from build123d import *

# Parameters (mm, degrees)
SKETCH1_R           = 52.3875
SKETCH1_R_2         = 50.8
BOSS_EXTRUDE1_DEPTH = 7.9
CUT_EXTRUDE1_START  = 3.95
SKETCH1_3_R         = 52.3875
SKETCH1_3_R_2       = 50.8
CUT_EXTRUDE1_DEPTH  = 1.7653


with BuildPart() as part:
    # Sketch1 → Boss-Extrude1 (new body)
    with BuildSketch(Plane(origin=(0, 0, 0), x_dir=(1, 0, 0), z_dir=(0, 1, 0))):
        with Locations(Location((0, 0, 0), (0, 0, 270))):
            Circle(SKETCH1_R)
        Circle(SKETCH1_R_2, mode=Mode.SUBTRACT)
        Circle(SKETCH1_R_2)
        with BuildLine():
            Line((-2.54, 4.028623369), (-2.54, 45.967377631))
            ThreePointArc((-2.54, 45.967377631), (-32.553428439, 32.553428439), (-45.967377631, 2.54))
            Line((-45.967377631, 2.54), (-4.028623369, 2.54))
            ThreePointArc((-4.028623369, 2.54), (-3.367596045, 3.367596045), (-2.54, 4.028623369))
        make_face(mode=Mode.SUBTRACT)
        with BuildLine():
            Line((4.028623369, 2.54), (45.967377631, 2.54))
            ThreePointArc((45.967377631, 2.54), (32.553428439, 32.553428439), (2.54, 45.967377631))
            Line((2.54, 45.967377631), (2.54, 4.028623369))
            ThreePointArc((2.54, 4.028623369), (3.367596045, 3.367596045), (4.028623369, 2.54))
        make_face(mode=Mode.SUBTRACT)
        with BuildLine():
            Line((2.54, -4.028623369), (2.54, -45.967377631))
            ThreePointArc((2.54, -45.967377631), (32.553428439, -32.553428439), (45.967377631, -2.54))
            Line((45.967377631, -2.54), (4.028623369, -2.54))
            ThreePointArc((4.028623369, -2.54), (3.367596045, -3.367596045), (2.54, -4.028623369))
        make_face(mode=Mode.SUBTRACT)
        with BuildLine():
            ThreePointArc((2.01246118, -1.8), (2.7, 0), (2.01246118, 1.8))
            Line((2.01246118, 1.8), (-2.01246118, 1.8))
            ThreePointArc((-2.01246118, 1.8), (-2.7, 0), (-2.01246118, -1.8))
            Line((-2.01246118, -1.8), (2.01246118, -1.8))
        make_face(mode=Mode.SUBTRACT)
        with BuildLine():
            ThreePointArc((-45.967377631, -2.54), (-32.553428439, -32.553428439), (-2.54, -45.967377631))
            Line((-2.54, -45.967377631), (-2.54, -4.028623369))
            ThreePointArc((-2.54, -4.028623369), (-3.367596045, -3.367596045), (-4.028623369, -2.54))
            Line((-4.028623369, -2.54), (-45.967377631, -2.54))
        make_face(mode=Mode.SUBTRACT)
    extrude(amount=BOSS_EXTRUDE1_DEPTH)

    # Sketch1<3> → Cut-Extrude1 (cut, symmetric)
    with BuildSketch(Plane(origin=(0, 0, 0), x_dir=(1, 0, 0), z_dir=(0, 1, 0)).offset(CUT_EXTRUDE1_START)):
        with Locations(Location((0, 0, 0), (0, 0, 270))):
            Circle(SKETCH1_3_R)
        with Locations(Location((0, 0, 0), (0, 0, 270))):
            Circle(SKETCH1_3_R_2, mode=Mode.SUBTRACT)
    extrude(amount=CUT_EXTRUDE1_DEPTH, both=True, mode=Mode.SUBTRACT)


solid = part.part
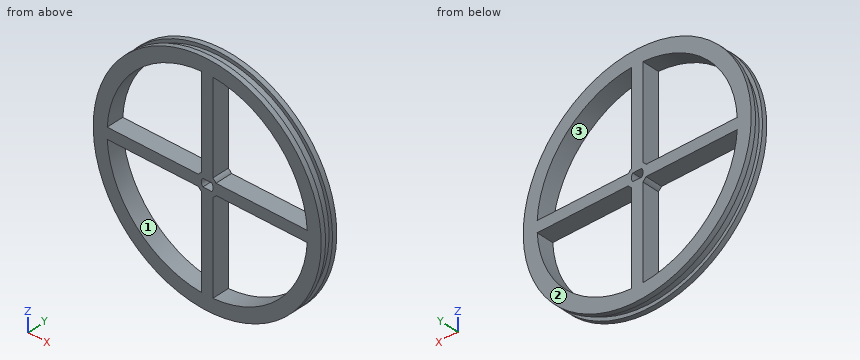
Read the model definition and answer for the solid it produces. Units are mm, in the model's axes. Face numbers are marked on the shaded views. Coordinates: 2 decimals unless noted, no trailing zeros. Write each loop counter-clockwise with the first axis right and the second up, starting at its lowest first coordinate (ties: lowest second). Pieces come first, ordered by that corner, then holes. Notation, with made-up numbers: M 89.25,-28.5 L 143.25,-28.5 A14 cw 143.25,-3.5 Z; hole C 63.5,-14 d8. An arc over 180 degrees is marked long. Use a Markdown table: item, result.
Q1. The part is cut by section C-C, the plane y = 4.25. Write down the section's boundary in (x, z) (1 decimal), then the cut area to 3 significant figures.
Answer block:
| item | result |
|---|---|
| outline | C 0,0 d101.6; hole M -46,-2.5 A46 ccw -2.5,-46 L -2.5,-4 A4.8 cw -4,-2.5 Z; hole M -46,2.5 L -4,2.5 A4.8 cw -2.5,4 L -2.5,46 A46 ccw Z; hole M -2,-1.8 L 2,-1.8 A2.7 ccw 2,1.8 L -2,1.8 A2.7 ccw Z; hole M 2.5,-46 A46 ccw 46,-2.5 L 4,-2.5 A4.8 cw 2.5,-4 Z; hole M 2.5,4 A4.8 cw 4,2.5 L 46,2.5 A46 ccw 2.5,46 Z |
| area | 2,350 mm2 |
Q2. Determine the mould class of the marked faces 1, 2 and 3 for opening direction Z: released by +Z, released by -Z, zero draft, split by the parting line, or undercut.
Answer block:
| item | result |
|---|---|
| face 1 | undercut |
| face 2 | zero draft |
| face 3 | undercut |
Q3. Each of these flat-tipped pins is pushed along its axis until it touches: pin 1 Ø3 at (x, y) = (0.5, 3.5) entering from -Z; pin 2 Ø3 at (y, z) = (2.5, -37.5) entering from +X; pin 3 Ø2.5 at (y, z) = (4, 25) entering from +X; pin 4 Ø1 at (y, z) = (3.5, -12.5) entering from +X. Where does it stop, or does it pass through?
Answer block:
| item | result |
|---|---|
| pin 1 | stops at z = -52.39 |
| pin 2 | stops at x = 38.03 |
| pin 3 | stops at x = 44.91 |
| pin 4 | stops at x = 49.36 |
Q4. The part is cut by section B-B, the plane x = 0. Write down the section's boundary in (y, z).
Answer block:
| item | result |
|---|---|
| outline | M 0,-52.39 L 2.18,-52.39 L 2.18,-50.8 L 5.72,-50.8 L 5.72,-52.39 L 7.9,-52.39 L 7.9,-1.8 L 0,-1.8 Z; M 0,1.8 L 7.9,1.8 L 7.9,52.39 L 5.72,52.39 L 5.72,50.8 L 2.18,50.8 L 2.18,52.39 L 0,52.39 Z |
Q5. The part is cut by section A-A, the plane z = 0. Write down the section's boundary in (x, y), then the cut area to 3 significant figures.
Answer block:
| item | result |
|---|---|
| outline | M -52.39,0 L -2.7,0 L -2.7,7.9 L -52.39,7.9 L -52.39,5.72 L -50.8,5.72 L -50.8,2.18 L -52.39,2.18 Z; M 2.7,0 L 52.39,0 L 52.39,2.18 L 50.8,2.18 L 50.8,5.72 L 52.39,5.72 L 52.39,7.9 L 2.7,7.9 Z |
| area | 774 mm2 |
Q6. Straight lines are drawn through the part: L1, parallel to X at y = 3.75, z = -16; L2, parallel to Z at x = -30.5, y = 7.5; L3, parallel to Z at x = 12, y = 7.5. For each, find the intervals that lie inside material, in ascending order. Write a range as [from, to].
Answer block:
| item | result |
|---|---|
| L1 | x = [-48.21, -43.17], [-2.54, 2.54], [43.17, 48.21] |
| L2 | z = [-42.59, -34.48], [-2.54, 2.54], [34.48, 42.59] |
| L3 | z = [-50.99, -44.45], [-2.54, 2.54], [44.45, 50.99] |
Q7. The part is cut by section D-D, the plane z = 33. Write down the section's boundary in (x, y).
Answer block:
| item | result |
|---|---|
| outline | M -40.69,0 L -32.1,0 L -32.1,7.9 L -40.69,7.9 L -40.69,5.72 L -38.62,5.72 L -38.62,2.18 L -40.69,2.18 Z; M -2.54,0 L 2.54,0 L 2.54,7.9 L -2.54,7.9 Z; M 32.1,0 L 40.69,0 L 40.69,2.18 L 38.62,2.18 L 38.62,5.72 L 40.69,5.72 L 40.69,7.9 L 32.1,7.9 Z |
